Verification items for the finished model (mm, model axes). A direction names the side the tool comes from. Coordinates: 2 decimals unless noted, no trailing zeros. Write each loop counter-clockwise with the first axis right and the second up, starting at its lowest first coordinate (ties: lowest second). Pieces come first, ordered by that corner, then holes. Notation, with made-up numbers: (42.5, -20.75) -> (51.5, -20.75) arc R16 ccw to (51.5, -7.75) -> close; hole circle Ø2 at (6.5, 36.25). An arc over 180 degrees is marked (long way). Use CSV: the item, a comma, the result in double quotes.
```python
from build123d import *

# Parameters (mm, degrees)
F1_DEPTH = 4
F2_R     = 5
F3_R     = 1


with BuildPart() as f1:
    # F0 (on Top) → F1 (new body)
    with BuildSketch(Plane.XY):
        with BuildLine():
            Line((5.846258, 15), (0, 0))
            Line((0, 0), (0, -2.497575))
            ThreePointArc((0, -2.497575), (0.487616, -2.985192), (0.975233, -2.497575))
            Line((0.975233, -2.497575), (9, -2.497575))
            Line((9, -2.497575), (9, -32.497575))
            Line((9, -32.497575), (0.975233, -32.497575))
            ThreePointArc((0.975233, -32.497575), (0.487616, -32.009959), (0, -32.497575))
            Line((0, -32.497575), (0, -36))
            Line((0, -36), (12, -36))
            Line((12, -36), (17.846258, 0))
            Line((17.846258, 0), (17.846258, 5.706935))
            Line((17.846258, 5.706935), (21.846258, 8.917766))
            Line((21.846258, 8.917766), (21.846258, 11.413869))
            ThreePointArc((21.846258, 11.413869), (21.746258, 11.513869), (21.646258, 11.413869))
            Line((21.646258, 11.413869), (17.846258, 11.413869))
            ThreePointArc((17.846258, 11.413869), (17.746258, 11.513869), (17.646258, 11.413869))
            Line((17.646258, 11.413869), (11.250778, 11.413869))
            ThreePointArc((11.250778, 11.413869), (11.150778, 11.513869), (11.050778, 11.413869))
            Line((11.050778, 11.413869), (8.426733, 11.413869))
            ThreePointArc((8.426733, 11.413869), (8.326733, 11.513869), (8.226733, 11.413869))
            Line((8.226733, 11.413869), (8.153742, 11.413869))
            Line((8.153742, 11.413869), (8.153742, 12.913869))
            Line((8.153742, 12.913869), (8.226733, 12.913869))
            ThreePointArc((8.226733, 12.913869), (8.326733, 12.813869), (8.426733, 12.913869))
            Line((8.426733, 12.913869), (11.050778, 12.913869))
            ThreePointArc((11.050778, 12.913869), (11.150778, 12.813869), (11.250778, 12.913869))
            Line((11.250778, 12.913869), (17.646258, 12.913869))
            ThreePointArc((17.646258, 12.913869), (17.746258, 12.813869), (17.846258, 12.913869))
            Line((17.846258, 12.913869), (21.646258, 12.913869))
            ThreePointArc((21.646258, 12.913869), (21.746258, 12.813869), (21.846258, 12.913869))
            Line((21.846258, 12.913869), (21.846258, 15))
            Line((21.846258, 15), (17.846258, 15))
            Line((17.846258, 15), (5.846258, 15))
        make_face()
    extrude(amount=F1_DEPTH)

    # F2
    f2_edges = [f1.edges().sort_by_distance(p)[0] for p in [
        (21.846258, 8.917766, 2),
        (17.846258, 5.706935, 2),
        (17.846258, 0, 2),
    ]]
    fillet(f2_edges, radius=F2_R)

    # F3
    f3_edges = [f1.edges().sort_by_distance(p)[0] for p in [
        (21.846258, 15, 2),
        (5.846258, 15, 2),
        (0, 0, 2),
        (12, -36, 2),
        (0, -36, 2),
    ]]
    fillet(f3_edges, radius=F3_R)


solid = f1.part
```
1) Cross-section at C-C (y = -11). Record the boundary of the cut face in (x, z).
Return value:
outline,"(9, 0) -> (16.06, 0) -> (16.06, 4) -> (9, 4) -> close"
2) Scan lines: L1, parallel to Y at x = 11, z = 0.25; L2, parallel to Y at x = 8.75, z = 3.6; L3, parallel to Y at x = 7, z = 2.15. Record each from-to range of solid material in increasing order.
Return value:
L1,"-36 to 11.41, 12.91 to 15"
L2,"-36 to -32.5, -2.5 to 11.41, 12.91 to 15"
L3,"-36 to -32.5, -2.5 to 15"
3) Cross-section at A-A (x = 9.5). Record the boundary of the cut face in (y, z).
Return value:
outline,"(-36, 0) -> (11.41, 0) -> (11.41, 4) -> (-36, 4) -> close; (12.91, 0) -> (15, 0) -> (15, 4) -> (12.91, 4) -> close"
4) Mould release check, pull along X, two halves, no side actions. Record for faces 3 (the flat face through (14, 12.914, 2)), 4 (the flat face through (21.846, 13.4, 2)), 5 (the flat face through (6, -36, 2)): released by +X, released by -X, zero draft, split by the parting line, or undercut.
Return value:
face 3,"undercut"
face 4,"released by +X"
face 5,"zero draft"
5) Gauge pin test, flat ends, axial feed: pin 1 (4 mm diameter, centred on x = 18.5, y = -12.5, fed in from +Z); pin 2 (1.5 mm diameter, centred on y = 2, z = 1, fed in from +X). Record the tip position at first contact, or that the pin passes through.
Return value:
pin 1,"through"
pin 2,"x = 17.85"
6) Cross-section at D-D (y = -25). Record the boundary of the cut face in (x, z).
Return value:
outline,"(9, 0) -> (13.79, 0) -> (13.79, 4) -> (9, 4) -> close"
7) Cross-section at B-B (x = 7). Record the boundary of the cut face in (y, z), plus the area to 3 significant figures.
Return value:
outline,"(-36, 0) -> (-32.5, 0) -> (-32.5, 4) -> (-36, 4) -> close; (-2.5, 0) -> (15, 0) -> (15, 4) -> (-2.5, 4) -> close"
area,"84.0 mm2"
8) Set-up check for faces 1 (the flat face through (20, 11.414, 2)), 2 (the flat face through (0, -1, 2)): record each of +Z, -Z, +X, -X, +Y, -Y from which the full face is reachable in a straight line by a thin tool's end or side.
Return value:
face 1,"+Z, -Z"
face 2,"+Z, -Z, -X, +Y, -Y"
